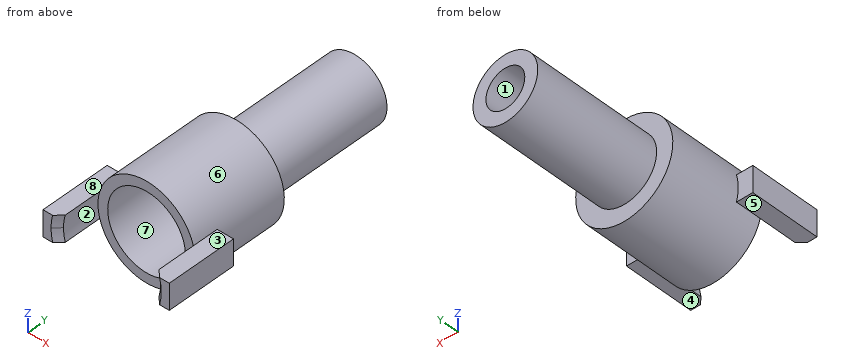
from build123d import *

# Parameters (mm, degrees)
PIN_R                     = 6.35
PIN_R_2                   = 3.81
BOSS_EXTRUDE4_DEPTH       = 25.4
HOLLOW_CYL_R              = 9.525
HOLLOW_CYL_R_2            = 7.62
BOSS_EXTRUDE5_DEPTH       = 19.05
SKETCH4_R                 = 7.62
BOSS_EXTRUDE7_DEPTH       = 2.54
BOSS_EXTRUDE9_DEPTH       = 7.62
BOSS_EXTRUDE9_2_DEPTH     = 7.62
BOSS_EXTRUDE10_DEPTH      = 8.636
BOSS_EXTRUDE10_DEPTH_BACK = 5.08
CHAMFER2_SIZE             = 1.27
CHAMFER4_SIZE             = 1.27


with BuildPart() as part:
    # Pin → Boss-Extrude4 (new body)
    with BuildSketch(Plane(origin=(0, 0, 0), x_dir=(1, 0, 0), z_dir=(0, 1, 0))):
        with Locations(Location((0, 0, 0), (0, 0, 270))):
            Circle(PIN_R)
        with Locations(Location((0, 0, 0), (0, 0, 270))):
            Circle(PIN_R_2, mode=Mode.SUBTRACT)
    extrude(amount=BOSS_EXTRUDE4_DEPTH)



with BuildPart() as body_2:
    # Hollow Cyl → Boss-Extrude5 (new body)
    with BuildSketch(Plane(origin=(0, 0, 0), x_dir=(1, 0, 0), z_dir=(0, 1, 0))):
        with Locations(Location((0, 0, 0), (0, 0, 270))):
            Circle(HOLLOW_CYL_R)
        with Locations(Location((0, 0, 0), (0, 0, 270))):
            Circle(HOLLOW_CYL_R_2, mode=Mode.SUBTRACT)
    extrude(amount=-BOSS_EXTRUDE5_DEPTH)


with BuildPart() as part_1:
    add(part.part)

    add(body_2.part)  # Boss-Extrude7 merges body 2
    # Sketch4 → Boss-Extrude7 (add)
    with BuildSketch(Plane(origin=(0, 0, 0), x_dir=(1, 0, 0), z_dir=(0, 1, 0))):
        with Locations(Location((0, 0, 0), (0, 0, 270))):
            Circle(SKETCH4_R)
    extrude(amount=-BOSS_EXTRUDE7_DEPTH)



with BuildPart() as body_2_2:
    # Sketch6 → Boss-Extrude9 (new body)
    with BuildSketch(Plane(origin=(0, -19.05, 0), x_dir=(-1, 0, 0), z_dir=(0, -1, 0))):
        with BuildLine():
            Line((9.180088507, -2.54), (12.3825, -2.54))
            Line((12.3825, -2.54), (12.3825, 2.54))
            Line((12.3825, 2.54), (9.180088507, 2.54))
            ThreePointArc((9.180088507, 2.54), (9.438378251, 1.281655564), (9.525, 0))
            ThreePointArc((9.525, 0), (9.438378251, -1.281655564), (9.180088507, -2.54))
        make_face()
    extrude(amount=BOSS_EXTRUDE9_DEPTH)


with BuildPart() as body_3:
    # Sketch6 → Boss-Extrude9 2 (new body)
    with BuildSketch(Plane(origin=(0, -19.05, 0), x_dir=(-1, 0, 0), z_dir=(0, -1, 0))):
        with BuildLine():
            Line((-12.3825, -2.54), (-9.180088507, -2.54))
            ThreePointArc((-9.180088507, -2.54), (-9.525, 0), (-9.180088507, 2.54))
            Line((-9.180088507, 2.54), (-12.3825, 2.54))
            Line((-12.3825, 2.54), (-12.3825, -2.54))
        make_face()
    extrude(amount=BOSS_EXTRUDE9_2_DEPTH)


with BuildPart() as part_2:
    add(part_1.part)

    add(body_2_2.part)  # Boss-Extrude10 merges body 2 2

    add(body_3.part)  # Boss-Extrude10 merges body 3
    # Sketch6_5 → Boss-Extrude10 (add, two sides: drawn at the far end of the back side and taken through both)
    with BuildSketch(Plane(origin=(0, -19.05, 0), x_dir=(-1, 0, 0), z_dir=(0, -1, 0)).offset(-BOSS_EXTRUDE10_DEPTH_BACK)):
        with BuildLine():
            Line((9.180088507, -2.54), (12.3825, -2.54))
            Line((12.3825, -2.54), (12.3825, 2.54))
            Line((12.3825, 2.54), (9.180088507, 2.54))
            ThreePointArc((9.180088507, 2.54), (9.438378251, 1.281655564), (9.525, 0))
            ThreePointArc((9.525, 0), (9.438378251, -1.281655564), (9.180088507, -2.54))
        make_face()
        with BuildLine():
            Line((-12.3825, -2.54), (-9.180088507, -2.54))
            ThreePointArc((-9.180088507, -2.54), (-9.525, 0), (-9.180088507, 2.54))
            Line((-9.180088507, 2.54), (-12.3825, 2.54))
            Line((-12.3825, 2.54), (-12.3825, -2.54))
        make_face()
    extrude(amount=BOSS_EXTRUDE10_DEPTH + BOSS_EXTRUDE10_DEPTH_BACK)

    # Chamfer2
    chamfer2_edges = [part_2.edges().sort_by_distance(p)[0] for p in [
        (9.525, -27.686, 0),
    ]]
    chamfer(chamfer2_edges, length=CHAMFER2_SIZE)

    # Chamfer4
    chamfer4_edges = [part_2.edges().sort_by_distance(p)[0] for p in [
        (-9.525, -27.686, 0),
    ]]
    chamfer(chamfer4_edges, length=CHAMFER4_SIZE)


solid = part_2.part
Can you work these out from the model? Positions are in its coordinate system, mm. Face numbers are marked on the shaded views. A direction names the side the tool comes from. Coordinates: 2 decimals unless noted, no trailing zeros. Order: outer loops, then holes, each group sorted by start corner. A loop starts at its lowest first (then second) coordinate and runs counter-clockwise, first axis right, second up. Notation, with made-up numbers: (57, -26) - (66, -26) arc R19 cw to (66, -6) - close; hole circle Ø8 at (-6.75, 67.25). An arc over 180 degrees is marked (long way). Answer as a JSON object with one key per item and string values. Group by question number.
Q1. Imagine slicing it at A-A (x = 0). Please give me the cut outline in (y, z) (3 decimals).
Q2. We'd pull the mould along X, two halves only. Please class the marked faces 6, 7 and 8: +X half, -X half, draft (parallel to the pull), parting line (faces both ways), or undercut.
Q3. Imagine slicing it at D-D (x = -2.5). Please give me the cut outline in (y, z).
Q4. I need wall thicknesses on line 1 (X direction, y = 9.5, z = 0); line 2 (Y direction, x = -3.75, z = 5); line 3 (Y direction, x = 4, z = -8.5). Which ranges of each line are inside material? Lowest first, please. Write a range as from..to.
Q5. Imagine slicing it at B-B (z = -4.75). Please give me the cut outline in (x, y).
Q6. Imagine slicing it at C-C (y = -0.5). Please give me the cut outline in (x, z) (3 decimals).
Q7. Will these pins go through, and if not, where does the flat tip stop? P1, Ø1, axis at x = -10.5, z = -0.5, coming from the +Y side; P2, Ø4, axis at y = 4.5, z = -4, coming from the +X side; P3, Ø1.5, axis at x = 3, y = 13, coming from the +Z side.
Q8. On a 3-axis mill with a long thin cutter (end or side, diameter ignored), from which of +Z, -Z, +X, -X, +Y, -Y can I reach the whole of each face in a straight line? I mean the marked faces 1, 2, 3, 4 and 5. Say none if no direction works.
Determined:
{
 "1": {"outline": "(-19.05, -9.525) - (0, -9.525) - (0, -6.35) - (25.4, -6.35) - (25.4, -3.81) - (0, -3.81) - (0, 3.81) - (25.4, 3.81) - (25.4, 6.35) - (0, 6.35) - (0, 9.525) - (-19.05, 9.525) - (-19.05, 7.62) - (-2.54, 7.62) - (-2.54, -7.62) - (-19.05, -7.62) - close"},
 "2": {"face 6": "parting line", "face 7": "undercut", "face 8": "draft"},
 "3": {"outline": "(-19.05, -9.19) - (0, -9.19) - (0, -5.84) - (25.4, -5.84) - (25.4, -2.88) - (0, -2.88) - (0, 2.88) - (25.4, 2.88) - (25.4, 5.84) - (0, 5.84) - (0, 9.19) - (-19.05, 9.19) - (-19.05, 7.2) - (-2.54, 7.2) - (-2.54, -7.2) - (-19.05, -7.2) - close"},
 "4": {"line 1": "x = -6.35..-3.81, 3.81..6.35", "line 2": "y = -2.54..25.4", "line 3": "y = -19.05..0"},
 "5": {"outline": "(-8.26, -19.05) - (-5.96, -19.05) - (-5.96, -2.54) - (5.96, -2.54) - (5.96, -19.05) - (8.26, -19.05) - (8.26, 0) - (4.21, 0) - (4.21, 25.4) - (-4.21, 25.4) - (-4.21, 0) - (-8.26, 0) - close"},
 "6": {"outline": "circle Ø19.05 at (0, 0)"},
 "7": {"P1": "stops at y = -13.97", "P2": "stops at x = 6.03", "P3": "stops at z = 5.94"},
 "8": {"face 1": "+Y", "face 2": "-Y", "face 3": "+Z, +X, +Y, -Y", "face 4": "-Z, +X, +Y, -Y", "face 5": "-Z, -X, +Y, -Y"}
}
